The listing builds one solid part. Answer for the finished solid, in the listing's coordinates (mm). A direction names the side the tool comes from. Round coordinates to 2 decimals unless told otherwise and drop trailing zeros. Order: outer loops, then holes, each group sorted by start corner. A loop starts at its lowest first (then second) coordinate and runs counter-clockwise, first axis right, second up. Notation, with made-up numbers: (-23, 47.25) -> (26, 47.25) arc R22 ccw to (26, 53.25) -> close; hole circle Ø6 at (80, 34.25). An arc over 180 degrees is marked (long way). Answer in a Markdown table with one row per item. Add a question column.
```python
from build123d import *

# Parameters (mm, degrees)
SKETCH1_W           = 100
SKETCH1_H           = 30
BOSS_EXTRUDE1_DEPTH = 5
SKETCH2_W           = 6
SKETCH2_H           = 50
BOSS_EXTRUDE2_DEPTH = 30
SKETCH3_W           = 6
SKETCH3_H           = 52.5
BOSS_EXTRUDE3_DEPTH = 50
SKETCH4_R           = 5
BOSS_EXTRUDE4_DEPTH = 20
CHAMFER1_SIZE       = 10
FILLET1_R           = 10
CHAMFER2_SIZE       = 10
FILLET2_R           = 4
SKETCH5_W           = 100
SKETCH5_H           = 5
BOSS_EXTRUDE5_DEPTH = 10
CHAMFER3_SIZE       = 10
SKETCH7_R           = 2.1
CUT_EXTRUDE1_DEPTH  = 137.587883796
CUT_EXTRUDE2_DEPTH  = 108.075907654
FILLET3_R           = 10
SKETCH9_R           = 6
BOSS_EXTRUDE6_DEPTH = 2
CHAMFER4_SIZE       = 0.5
CUT_EXTRUDE3_START  = 1
SKETCH10_R          = 5
SKETCH10_R_2        = 4
CUT_EXTRUDE3_DEPTH  = 1
CHAMFER5_SIZE       = 0.5


with BuildPart() as part:
    # Sketch1 → Boss-Extrude1 (new body)
    with BuildSketch(Plane.XY):
        with Locations((50, 15)):
            Rectangle(SKETCH1_W, SKETCH1_H)
    extrude(amount=BOSS_EXTRUDE1_DEPTH)

    # Sketch2 → Boss-Extrude2 (add)
    with BuildSketch(Plane(origin=(0, 30, 0), x_dir=(1, 0, 0), z_dir=(0, 1, 0))):
        with Locations((50, 22.5)):
            Rectangle(SKETCH2_W, SKETCH2_H)
    extrude(amount=-BOSS_EXTRUDE2_DEPTH)

    # Sketch3 → Boss-Extrude3 (add)
    with BuildSketch(Plane(origin=(0, 30, 0), x_dir=(1, 0, 0), z_dir=(0, 1, 0))):
        with Locations((50, 21.25)):
            Rectangle(SKETCH3_W, SKETCH3_H)
    extrude(amount=BOSS_EXTRUDE3_DEPTH)

    # Sketch4 → Boss-Extrude4 (add)
    with BuildSketch(Plane.ZY.offset(-47)):
        with Locations((-40, 74)):
            Circle(SKETCH4_R)
    extrude(amount=BOSS_EXTRUDE4_DEPTH)

    # Chamfer1
    chamfer1_edges = [part.edges().sort_by_distance(p)[0] for p in [
        (50, 0, -47.5),
    ]]
    chamfer(chamfer1_edges, length=CHAMFER1_SIZE)

    # Fillet1
    fillet1_edges = [part.edges().sort_by_distance(p)[0] for p in [
        (50, 80, 5),
        (50, 80, -47.5),
    ]]
    fillet(fillet1_edges, radius=FILLET1_R)

    # Chamfer2
    chamfer2_edges = [part.edges().sort_by_distance(p)[0] for p in [
        (47, 30, 2.5),
        (53, 30, 2.5),
    ]]
    chamfer(chamfer2_edges, length=CHAMFER2_SIZE)

    # Fillet2
    fillet2_edges = [part.edges().sort_by_distance(p)[0] for p in [
        (0, 0, 2.5),
        (100, 0, 2.5),
        (100, 30, 2.5),
        (0, 30, 2.5),
    ]]
    fillet(fillet2_edges, radius=FILLET2_R)

    # Sketch5 → Boss-Extrude5 (add)
    with BuildSketch(Plane(origin=(0, 0, 0), x_dir=(-1, 0, 0), z_dir=(0, 0, -1))):
        with Locations((-50, 15)):
            Rectangle(SKETCH5_W, SKETCH5_H)
    extrude(amount=BOSS_EXTRUDE5_DEPTH)

    # Chamfer3
    chamfer3_edges = [part.edges().sort_by_distance(p)[0] for p in [
        (0, 15, -10),
        (100, 15, -10),
    ]]
    chamfer(chamfer3_edges, length=CHAMFER3_SIZE)

    # Sketch7 → Cut-Extrude1 (cut, through all)
    with BuildSketch(Plane(origin=(0, 0, 0), x_dir=(-1, 0, 0), z_dir=(0, 0, -1))):
        with Locations((-92, 24)):
            Circle(SKETCH7_R)
        with Locations((-8, 24)):
            Circle(SKETCH7_R)
        with Locations((-8, 6)):
            Circle(SKETCH7_R)
        with Locations((-92, 6)):
            Circle(SKETCH7_R)
    extrude(amount=-CUT_EXTRUDE1_DEPTH, mode=Mode.SUBTRACT)

    # Sketch8 → Cut-Extrude2 (cut, through all)
    with BuildSketch(Plane.ZY.offset(-47)):
        with BuildLine():
            Line((-36.644039957, 77.706417703), (5, 40))
            Line((5, 40), (5, 70))
            ThreePointArc((5, 70), (2.071067812, 77.071067812), (-5, 80))
            Line((-5, 80), (-37.5, 80))
            ThreePointArc((-37.5, 80), (-44.571067812, 77.071067812), (-47.5, 70))
            Line((-47.5, 70), (-47.5, 10))
            Line((-47.5, 10), (-44.996201229, 74.194867332))
            ThreePointArc((-44.996201229, 74.194867332), (-41.937871072, 78.609192522), (-36.644039957, 77.706417703))
        make_face()
    extrude(amount=-CUT_EXTRUDE2_DEPTH, mode=Mode.SUBTRACT)

    # Fillet3
    fillet3_edges = [part.edges().sort_by_distance(p)[0] for p in [
        (50, 40, 5),
        (50, 0, -37.5),
        (50, 10, -47.5),
    ]]
    fillet(fillet3_edges, radius=FILLET3_R)

    # Sketch9 → Boss-Extrude6 (add)
    with BuildSketch(Plane.ZY.offset(-47)):
        with Locations(Location((-40, 74, 0), (0, 0, 211.323728943))):
            Circle(SKETCH9_R)
    extrude(amount=BOSS_EXTRUDE6_DEPTH)

    # Chamfer4
    chamfer4_edges = [part.edges().sort_by_distance(p)[0] for p in [
        (27, 74, -45),
    ]]
    chamfer(chamfer4_edges, length=CHAMFER4_SIZE)

    # Sketch10 → Cut-Extrude3 (cut)
    with BuildSketch(Plane.ZY.offset(-30).offset(CUT_EXTRUDE3_START)):
        with Locations((-40, 74)):
            Circle(SKETCH10_R)
        with Locations((-40, 74)):
            Circle(SKETCH10_R_2, mode=Mode.SUBTRACT)
    extrude(amount=-CUT_EXTRUDE3_DEPTH, mode=Mode.SUBTRACT)

    # Chamfer5
    chamfer5_edges = [part.edges().sort_by_distance(p)[0] for p in [
        (29, 74, -45),
        (30, 74, -45),
    ]]
    chamfer(chamfer5_edges, length=CHAMFER5_SIZE)


solid = part.part
```
Item 1: Find the intervals of material crossed by probe 1 along Y at (x, z) = (8, 1.6); probe 2 along X at (y, z) = (12.5, -14.5); probe 3 along Z at (x, y) = (7, 26), in increasing order. Write a range as [from, to].
Item 2: Flat-ended cylindrical pins translate along their axes: P1, Ø10, axis at x = 23, y = 71.5, coming from the -Z side; P2, Ø5, axis at x = 32, z = -7, coming from the -Y side; P3, Ø4, axis at x = 49, z = -40, coming from the -Y side. Find the tip coordinate at first contact, or state that the pin passes through.
Item 3: The part is cut by section D-D, the plane z = -14. Give the vertices of the cut face in (x, y), and give its area (3 significant figures).
Item 4: For a pull along Y with two mould halves and no side action, classify faces 1 (the face through (50, 0, -1)), 2 (the face through (94.1, 24.09, 2.46)), 3 (the face through (49, 18, 5)), 4 (the face through (9.548, 25.419, 2.465)) as released by +Y, released by -Y, zero draft, split by the parting line, or undercut.
Item 5: The part is cut by section C-C, the plane x = 68.5. Give the vertices of the cut face in (y, z).
Item 6: The part is cut by section B-B, the plane y = 24. Give the vertices of the cut face in (x, z), and give its area (3 significant figures).
Item 7: A tool of negligible diameter and unlimited length cuts with its end or side. For faces 5 (the face through (72, 15, -10)), 6 (the face through (76, 24, 0)), 7 (the face through (23, 24, 0)), 8 (the face through (23, 6, 0)), 9 (the face through (29.493, 70.095, -40.867)), from which of +Z, -Z, +X, -X, +Y, -Y can it reach the whole face along a straight path? Write none if from no direction.
Item 8: The part is cut by section A-A, the plane x = 8. Give the vertices of the cut face in (y, z).
Resolved:
| question | item | result |
|---|---|---|
| 1 | probe 1 | [0, 3.9], [8.1, 21.9], [26.1, 30] |
| 1 | probe 2 | [47, 53] |
| 1 | probe 3 | [0, 5] |
| 2 | P1 | z = -44.99 |
| 2 | P2 | y = 12.5 |
| 2 | P3 | y = 1.14 |
| 3 | outline | (47, 0) -> (53, 0) -> (53, 57.2) -> (47, 57.2) -> close |
| 3 | area | 343 mm2 |
| 4 | face 1 | released by -Y |
| 4 | face 2 | undercut |
| 4 | face 3 | zero draft |
| 4 | face 4 | undercut |
| 5 | outline | (0, 0) -> (12.5, 0) -> (12.5, -10) -> (17.5, -10) -> (17.5, 0) -> (30, 0) -> (30, 5) -> (0, 5) -> close |
| 6 | outline | (0, 0) -> (5.9, 0) -> (5.9, 5) -> (0, 5) -> close; (10.1, 0) -> (47, 0) -> (47, -46.95) -> (53, -46.95) -> (53, 0) -> (89.9, 0) -> (89.9, 5) -> (10.1, 5) -> close; (94.1, 0) -> (100, 0) -> (100, 5) -> (94.1, 5) -> close |
| 6 | area | 740 mm2 |
| 7 | face 5 | -Z, +X, +Y, -Y |
| 7 | face 6 | -Z, +X, +Y |
| 7 | face 7 | -Z, -X, +Y |
| 7 | face 8 | -Z, -X, -Y |
| 7 | face 9 | none |
| 8 | outline | (0, 0) -> (3.9, 0) -> (3.9, 5) -> (0, 5) -> close; (8.1, 0) -> (12.5, 0) -> (12.5, -8) -> (17.5, -8) -> (17.5, 0) -> (21.9, 0) -> (21.9, 5) -> (8.1, 5) -> close; (26.1, 0) -> (30, 0) -> (30, 5) -> (26.1, 5) -> close |
